from build123d import *

# Parameters (mm, degrees)
SKETCH1_R           = 19
BOSS_EXTRUDE1_DEPTH = 203
SKETCH2_R           = 12.5
SKETCH2_R_2         = 10
BOSS_EXTRUDE2_DEPTH = 15
BOSS_EXTRUDE3_START = 15
SKETCH3_R           = 12.5
SKETCH3_R_2         = 10
BOSS_EXTRUDE3_DEPTH = 15


with BuildPart() as part:
    # Sketch1 → Boss-Extrude1 (new body)
    with BuildSketch(Plane(origin=(0, 0, 0), x_dir=(1, 0, 0), z_dir=(0, 1, 0))):
        with Locations(Location((0, 0, 0), (0, 0, 90))):
            Circle(SKETCH1_R)
    extrude(amount=BOSS_EXTRUDE1_DEPTH)

    # Sketch2 → Boss-Extrude2 (add)
    with BuildSketch(Plane.XZ):
        with Locations(Location((0, 0, 0), (0, 0, 90))):
            Circle(SKETCH2_R)
        with Locations(Location((0, 0, 0), (0, 0, 270))):
            Circle(SKETCH2_R_2, mode=Mode.SUBTRACT)
    extrude(amount=BOSS_EXTRUDE2_DEPTH)

    # Sketch3 → Boss-Extrude3 (add)
    with BuildSketch(Plane(origin=(0, 203, 0), x_dir=(1, 0, 0), z_dir=(0, 1, 0)).offset(BOSS_EXTRUDE3_START)):
        with Locations(Location((0, 0, 0), (0, 0, 270))):
            Circle(SKETCH3_R)
        with Locations(Location((0, 0, 0), (0, 0, 90))):
            Circle(SKETCH3_R_2, mode=Mode.SUBTRACT)
    extrude(amount=-BOSS_EXTRUDE3_DEPTH)


solid = part.part
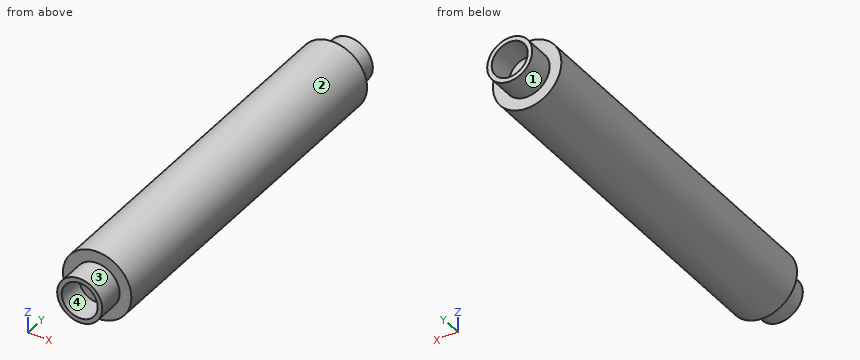
CAD build for the part. Positions are in the model's coordinates, mm. Face numbers are marked on the shaded views. A direction names the side the tool comes from. Round coordinates to 2 decimals unless told otherwise and drop trailing zeros. Write each loop counter-clockwise with the first axis right and the second up, starting at its lowest first coordinate (ties: lowest second). Pieces come first, ordered by that corner, then holes. Notation, with made-up numbers: M -33.75,-6 L -25.75,-6 A20 cw -25.75,8 Z; hole C -27.75,-19 d4. An arc over 180 degrees is marked long. Use a Markdown table: item, result. Add a question column.
1. Slice it at C-C on y = 105.5. Give the cut face in (x, z), then the cut area to 3 significant figures.
2. Flat gauge pins, fed straight in: P1, Ø1.5, axis at x = -13.5, z = -6, coming from the +Y side; P2, Ø18, axis at x = 0, z = 0, coming from the -Y side; P3, Ø10, axis at y = 142.5, z = 3, coming from the +X side; P4, Ø22, axis at x = -1, z = 4, coming from the -Y side. Where does each tip first touch, or does it go through?
3. Drill centre lines: probe 1 along X at (y, z) = (207, 0); probe 2 along X at (y, z) = (-1.5, 2); probe 3 along Y at (x, z) = (-16, -4). Where is each one in solid material? Low to high.
4. 3-axis set-ups, long thin cutter, end or side, ignore diameter. For the marked faces 1 and 2: which of +Z, -Z, +X, -X, +Y, -Y reach the whole face in a straight line?
5. Pull direction X, two halves, no side cores. Call the marked faces 3 and 4: released by +X, released by -X, zero draft, split by the parting line, or undercut.
6. Slice it at A-A on z = 0. Give the cut face in (x, y), then the cut area to 3 significant figures.
7. Slice it at D-D on z = 16.5. Give the cut face in (x, y).
8. Slice it at B-B on x = 0. Give the cut face in (y, z).
Reply:
| question | item | result |
|---|---|---|
| 1 | outline | C 0,0 d38 |
| 1 | area | 1,130 mm^2 |
| 2 | P1 | stops at y = 203 |
| 2 | P2 | stops at y = 0 |
| 2 | P3 | stops at x = 19 |
| 2 | P4 | stops at y = -15 |
| 3 | probe 1 | x = -12.5 to -10, 10 to 12.5 |
| 3 | probe 2 | x = -12.34 to -9.8, 9.8 to 12.34 |
| 3 | probe 3 | y = 0 to 203 |
| 4 | face 1 | +Y |
| 4 | face 2 | +Y, -Y |
| 5 | face 3 | split by the parting line |
| 5 | face 4 | undercut |
| 6 | outline | M -19,0 L -12.5,0 L -12.5,-15 L -10,-15 L -10,0 L 10,0 L 10,-15 L 12.5,-15 L 12.5,0 L 19,0 L 19,203 L 12.5,203 L 12.5,218 L 10,218 L 10,203 L -10,203 L -10,218 L -12.5,218 L -12.5,203 L -19,203 Z |
| 6 | area | 7,860 mm^2 |
| 7 | outline | M -9.42,0 L 9.42,0 L 9.42,203 L -9.42,203 Z |
| 8 | outline | M -15,-12.5 L 0,-12.5 L 0,-19 L 203,-19 L 203,-12.5 L 218,-12.5 L 218,-10 L 203,-10 L 203,10 L 218,10 L 218,12.5 L 203,12.5 L 203,19 L 0,19 L 0,12.5 L -15,12.5 L -15,10 L 0,10 L 0,-10 L -15,-10 Z |
